```python
from build123d import *

# Parameters (mm, degrees)
F2_SIZE = 0.5
F3_R    = 1


with BuildPart() as f1:
    # F0 (on Front) → F1 (revolve)
    with BuildSketch(Plane.XZ):
        Polygon((-44.45, 35), (-44.45, 28.575), (107.95, 28.575), (107.95, 38.1), (0, 38.1), (0, 44.45), (-15.875, 44.45), (-15.875, 35), (-35.95, 35), (-35.95, 33.2), (-38.5, 33.2), (-38.5, 35), align=None)
    revolve(axis=Axis((19.276485, 0, 0), (1, 0, 0)))

    # F2
    f2_edges = [f1.edges().sort_by_distance(p)[0] for p in [
        (107.95, 0, -38.1),
        (107.95, 0, -28.575),
        (-44.45, 0, -28.575),
        (-44.45, 0, -35),
        (-15.875, 0, -44.45),
        (0, 0, -44.45),
    ]]
    chamfer(f2_edges, length=F2_SIZE)

    # F3
    f3_edges = [f1.edges().sort_by_distance(p)[0] for p in [
        (-15.875, 0, -35),
        (0, 0, -38.1),
    ]]
    fillet(f3_edges, radius=F3_R)


solid = f1.part
```
Can you work these out from the model? Positions are in its coordinate system, mm. A direction names the side the tool comes from. Give positions to 0.01 mm unless a question says otherwise; leave off trailing zeros. Order: outer loops, then holes, each group sorted by start corner. A loop starts at its lowest first (then second) coordinate and runs counter-clockwise, first axis right, second up. Notation, with made-up numbers: (-34.75, 23) - (-25.75, 23) arc R10 ccw to (-25.75, 32) - close; hole circle Ø11 at (24, -3.5). An arc over 180 degrees is marked (long way). Use a Markdown table: item, result. Add a question column.
Q1. I'm going to push flat-ended pins straight in: pin 1 (1 mm diameter, centred on x = 33.5, y = -31, fed in from +Z); pin 2 (6 mm diameter, centred on x = 37.5, y = 30.5, fed in from -Z); pin 3 (10 mm diameter, centred on x = 15.5, z = 6, fed in from -Y). Where does each tip first touch, or does it pass through?
Q2. If we section it at A-A on x = -10: Write out the boundary of the cut face in (y, z) (3 decimals), plus the area to 3 significant figures.
Q3. If we mould it in two halves opening along Z, with no side actions, what happens to faces 4 (the cylindrical face through (32.81, -1.256, -28.547)), 5 (the flat face through (-35.95, -26, 21)), 6 (the cylindrical face through (53.48, 23.183, -30.235))? For each: released by +Z, released by -Z, zero draft, split by the parting line, or undercut.
Q4. On a 3-axis mill with a long thin cutter (end or side, diameter ignored), from which of +Z, -Z, +X, -X, +Y, -Y can I reach the whole of each face in a straight line? I mean faces 1 (the flat face through (-38.5, -26, -21)), 2 (the flat face through (0, 26, 30)), 3 (the flat face through (-15.875, 32.4, -16.5)). Say none if no direction works.
Q5. Please list where these lines run through material, in increasing order: line 1 along Y through (x, z) = (14.5, 0) (3 decimals); line 2 along Y through (x, z) = (-24, -1).
Q6. If we section it at B-B on x = 18.5: Write out the boundary of the cut face in (y, z) (3 decimals).
Answers follow:
| question | item | result |
|---|---|---|
| 1 | pin 1 | stops at z = 22.83 |
| 1 | pin 2 | stops at z = -26.37 |
| 1 | pin 3 | stops at y = -38.09 |
| 2 | outline | circle Ø88.9 at (0, 0); hole circle Ø57.15 at (0, 0) |
| 2 | area | 3,640 mm^2 |
| 3 | face 4 | undercut |
| 3 | face 5 | zero draft |
| 3 | face 6 | split by the parting line |
| 4 | face 1 | none |
| 4 | face 2 | +X |
| 4 | face 3 | -X |
| 5 | line 1 | y = -38.1 to -28.575, 28.575 to 38.1 |
| 5 | line 2 | y = -34.99 to -28.56, 28.56 to 34.99 |
| 6 | outline | circle Ø76.2 at (0, 0); hole circle Ø57.15 at (0, 0) |
